Model file for the job. Use its own axes, mm. Coordinates: 2 decimals unless noted, no trailing zeros. Write each loop counter-clockwise with the first axis right and the second up, starting at its lowest first coordinate (ties: lowest second). Pieces come first, ordered by that corner, then holes. Notation, with made-up numbers: (45, -36) - (101, -36) arc R29 ccw to (101, -5) - close; hole circle Ø6 at (-35.5, 49.25). An arc over 180 degrees is marked (long way). Put each result on its own line as item: value. Start each with the question number.
1. Drill centre lines: L1, parallel to Z at x = -0.25, y = -22.5; L2, parallel to Z at x = 5.5, y = -2.25; L3, parallel to X at y = -21.25, z = -4.5. Where is each one in solid material? Low to high. Write a range as from..to.
2. Saw through at A-A, the plane y = -2.25. Write the cut outline in (x, z), plus the area to 3 significant figures.
3. Drop flat-ended pins along their axis: P1, Ø2, axis at x = -1.5, y = -17, coming from the +Z side; P2, Ø1.5, axis at y = -16, z = -5, coming from the -X side; P3, Ø1.5, axis at y = -7.5, z = -3.5, coming from the -X side. Give the stop position or say it passes through.
```python
from build123d import *

# Parameters (mm, degrees)
F0_R     = 6.35
F1_DEPTH = 25.4
F2_SIZE  = 1.27
F3_SIZE  = 1.27


with BuildPart() as f1:
    # F0 (on Front) → F1 (new body)
    with BuildSketch(Plane.XZ):
        Circle(F0_R)
    extrude(amount=F1_DEPTH)

    # F2
    f2_edges = [f1.edges().sort_by_distance(p)[0] for p in [
        (-6.35, -25.4, 0),
    ]]
    chamfer(f2_edges, length=F2_SIZE)

    # F3
    f3_edges = [f1.edges().sort_by_distance(p)[0] for p in [
        (-6.35, 0, 0),
    ]]
    chamfer(f3_edges, length=F3_SIZE)


solid = f1.part
```
Final values:
1. L1: z = -6.35..6.35
1. L2: z = -3.17..3.17
1. L3: x = -4.48..4.48
2. outline: circle Ø12.7 at (0, 0)
2. area: 127 mm²
3. P1: stops at z = 6.33
3. P2: stops at x = -4.72
3. P3: stops at x = -5.72
